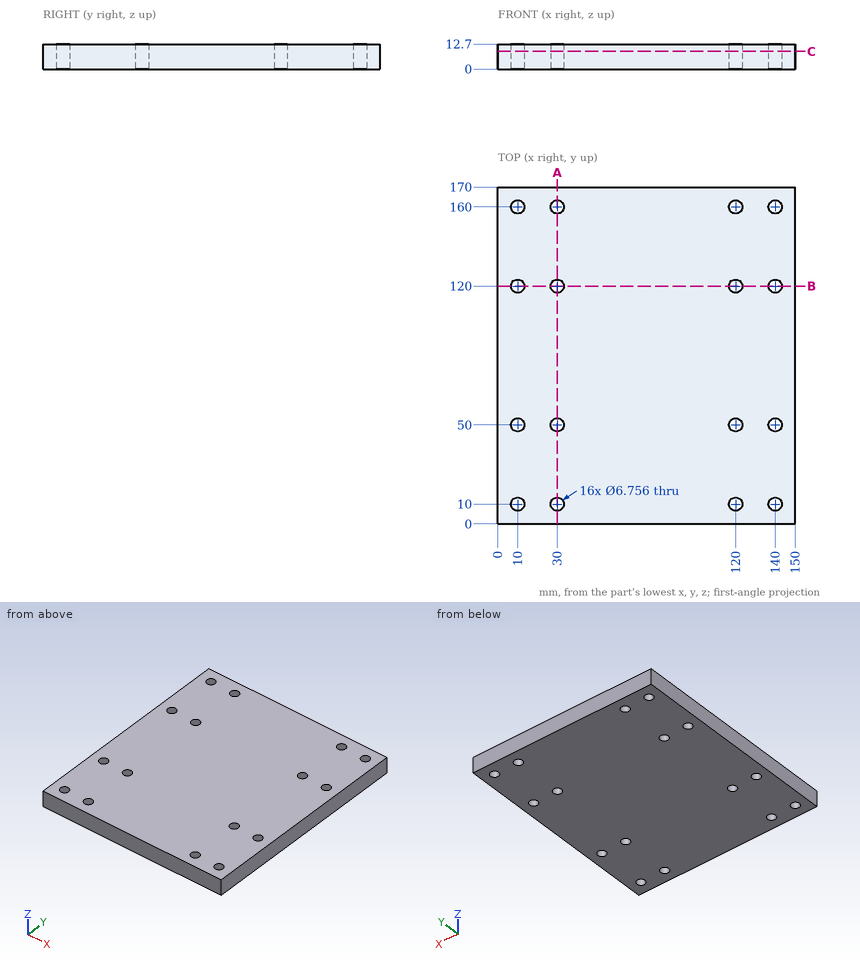
Job drawing, mm, ordinate dimensions from the low corner. One solid piece. Round coordinates to 2 decimals unless told otherwise and drop trailing zeros. Write each loop counter-clockwise with the first axis right and the second up, starting at its lowest first coordinate (ties: lowest second). Pieces come first, ordered by that corner, then holes. Notation, with made-up numbers: (66, 78) -> (74, 78) arc R16 cw to (74, 106) -> close; hole circle Ø5 at (-36.75, 35.5). An arc over 180 degrees is marked (long way). Answer as a JSON object with one key per item and string values.
(1) Band-saw the part on C-C, the plane z = 9. Count the separate pieces of the cut face and the enclosed holes in it, then the cut area to 3 significant figures.
Reported:
{"separate pieces": "1", "enclosed holes": "16", "area": "24,900 mm^2"}
(2) Band-saw the part on A-A, the plane x = 30. List the corners of the cut face in (y, z).
Reported:
{"outline": "(0, 0) -> (6.62, 0) -> (6.62, 12.7) -> (0, 12.7) -> close; (13.38, 0) -> (46.62, 0) -> (46.62, 12.7) -> (13.38, 12.7) -> close; (53.38, 0) -> (116.62, 0) -> (116.62, 12.7) -> (53.38, 12.7) -> close; (123.38, 0) -> (156.62, 0) -> (156.62, 12.7) -> (123.38, 12.7) -> close; (163.38, 0) -> (170, 0) -> (170, 12.7) -> (163.38, 12.7) -> close"}
(3) Band-saw the part on B-B, the plane y = 120. List the corners of the cut face in (x, z), then the cut area to 3 significant figures.
Reported:
{"outline": "(0, 0) -> (6.62, 0) -> (6.62, 12.7) -> (0, 12.7) -> close; (13.38, 0) -> (26.62, 0) -> (26.62, 12.7) -> (13.38, 12.7) -> close; (33.38, 0) -> (116.62, 0) -> (116.62, 12.7) -> (33.38, 12.7) -> close; (123.38, 0) -> (136.62, 0) -> (136.62, 12.7) -> (123.38, 12.7) -> close; (143.38, 0) -> (150, 0) -> (150, 12.7) -> (143.38, 12.7) -> close", "area": "1,560 mm^2"}
(4) Pin check, flat tip, straight feed: P1, Ø11, axis at x = 30, y = 160, coming from the -Z side. Stop position of the tip, or through.
Reported:
{"P1": "stops at z = 0"}
(5) Probe probe 1 along Y at (x, z) = (30, 4); probe 2 along X at (y, z) = (160, 9); probe 3 along X at (y, z) = (7.5, 4.25). List the from-to ranges inside material, lowest first. Write a range as [from, to].
Reported:
{"probe 1": "y = [0, 6.62], [13.38, 46.62], [53.38, 116.62], [123.38, 156.62], [163.38, 170]", "probe 2": "x = [0, 6.62], [13.38, 26.62], [33.38, 116.62], [123.38, 136.62], [143.38, 150]", "probe 3": "x = [0, 7.73], [12.27, 27.73], [32.27, 117.73], [122.27, 137.73], [142.27, 150]"}
